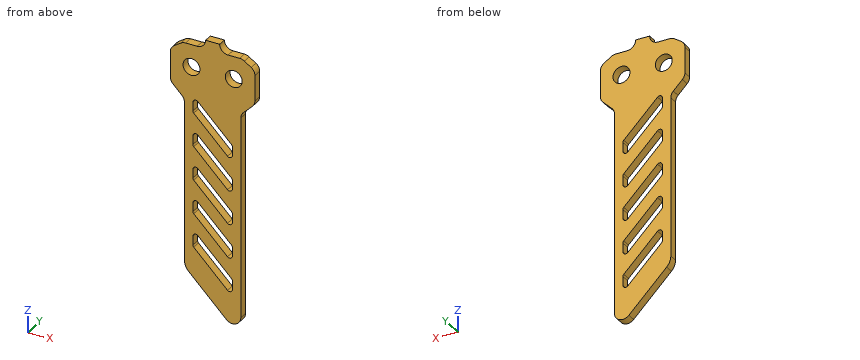
```python
from build123d import *
from OCP.BRepFilletAPI import BRepFilletAPI_MakeFillet

# Parameters (mm, degrees)
BOSS_EXTRUDE1_DEPTH     = 1.5
CUT_EXTRUDE1_DEPTH      = 105.097310244
CUT_EXTRUDE2_DEPTH      = 105.097310244
CUT_EXTRUDE2_DEPTH_BACK = 105.097310244
SKETCH2_R               = 3
FILLET1_R               = 3
FILLET2_R               = 3
FILLET3_R1              = 5
FILLET3_R2              = 3
FILLET4_R               = 1
LPATTERN1_COUNT         = 5
LPATTERN1_PITCH         = 12
FILLET4_OF_LPATTERN1_R  = 1


with BuildPart() as part:
    # Sketch1 → Boss-Extrude1 (new, symmetric)
    with BuildSketch(Plane(origin=(0, 0, 0), x_dir=(1, 0, 0), z_dir=(0, 1, 0))):
        Polygon((-10, 83), (10, 103), (10, 23), (15, 18), (15, 6), (10.5, 3), (2.5, 3), (2.5, 0), (-2.5, 0), (-2.5, 3), (-10.5, 3), (-15, 6), (-15, 18), (-10, 23), align=None)
    extrude(amount=BOSS_EXTRUDE1_DEPTH, both=True)

    # Sketch1<3> → Cut-Extrude1 (cut, symmetric)
    with BuildSketch(Plane(origin=(0, 0, 0), x_dir=(1, 0, 0), z_dir=(0, 1, 0))):
        Polygon((7, 89), (-7, 75), (-7, 69), (7, 83), align=None)
    cut_extrude1 = extrude(amount=CUT_EXTRUDE1_DEPTH, both=True, mode=Mode.SUBTRACT)

    # Sketch2 → Cut-Extrude2 (cut, two sides: drawn at the far end of the back side and taken through both)
    with BuildSketch(Plane(origin=(0, 0, 0), x_dir=(1, 0, 0), z_dir=(0, 1, 0)).offset(-CUT_EXTRUDE2_DEPTH_BACK)):
        with Locations(Location((-7.5, 11, 0), (0, 0, 270))):
            Circle(SKETCH2_R)
        with Locations(Location((7.5, 11, 0), (0, 0, 270))):
            Circle(SKETCH2_R)
    extrude(amount=CUT_EXTRUDE2_DEPTH + CUT_EXTRUDE2_DEPTH_BACK, mode=Mode.SUBTRACT)

    # Fillet1
    fillet1_edges = [part.edges().sort_by_distance(p)[0] for p in [
        (2.5, 0, -3),
        (-2.5, 0, -3),
    ]]
    fillet(fillet1_edges, radius=FILLET1_R - 0.0001)  # a hair under: the kernel refuses the full size

    # Fillet2
    fillet2_edges = [part.edges().sort_by_distance(p)[0] for p in [
        (-10, 0, -23),
        (-15, 0, -18),
        (-15, 0, -6),
        (-10.5, 0, -3),
        (10.5, 0, -3),
        (15, 0, -6),
        (15, 0, -18),
        (10, 0, -23),
    ]]
    fillet(fillet2_edges, radius=FILLET2_R)

    # Fillet3: one fillet with a radius per group of edges: ONE call of the kernel's fillet builder (fillet() takes one radius for all edges)
    fillet3_edges_1 = [part.edges().sort_by_distance(p)[0] for p in [
        (-10, 0, -83),
    ]]
    fillet3_edges_2 = [part.edges().sort_by_distance(p)[0] for p in [
        (10, 0, -103),
    ]]
    fillet3 = BRepFilletAPI_MakeFillet(part.part.solid().wrapped)
    for e in fillet3_edges_1:
        fillet3.Add(FILLET3_R1, e.wrapped)
    for e in fillet3_edges_2:
        fillet3.Add(FILLET3_R2, e.wrapped)
    add(Compound.cast(fillet3.Shape()), mode=Mode.REPLACE)

    # Fillet4
    fillet4_edges = [part.edges().sort_by_distance(p)[0] for p in [
        (-7, 0, -69),
        (-7, 0, -75),
        (7, 0, -89),
        (7, 0, -83),
    ]]
    fillet(fillet4_edges, radius=FILLET4_R)

    # LPattern1: Cut-Extrude1 ×5
    with Locations(*[(0, 0, i * LPATTERN1_PITCH) for i in range(1, LPATTERN1_COUNT)]):
        add(cut_extrude1, mode=Mode.SUBTRACT)

    # Fillet4 of LPattern1
    fillet4_of_lpattern1_edges = [part.edges().sort_by_distance(p)[0] for p in [
        (-7, 0, -57),
        (-7, 0, -63),
        (7, 0, -77),
        (7, 0, -71),
        (-7, 0, -45),
        (-7, 0, -51),
        (7, 0, -65),
        (7, 0, -59),
        (-7, 0, -33),
        (-7, 0, -39),
        (7, 0, -53),
        (7, 0, -47),
        (-7, 0, -21),
        (-7, 0, -27),
        (7, 0, -41),
        (7, 0, -35),
    ]]
    fillet(fillet4_of_lpattern1_edges, radius=FILLET4_OF_LPATTERN1_R)


solid = part.part
```
Build history of the part. All positions in model axes, mm. Round coordinates to 2 decimals unless told otherwise and drop trailing zeros. Order: outer loops, then holes, each group sorted by start corner. A loop starts at its lowest first (then second) coordinate and runs counter-clockwise, first axis right, second up. Notation, with made-up numbers: (45, -26.5) -> (69, -26.5) arc R23 ccw to (69, -3.5) -> close; hole circle Ø10 at (79.5, -27). An arc over 180 degrees is marked (long way). Answer in a Markdown table with one row per item.
1) Band-saw the part on D-D on y = -0.75. Give the number of separate pieces and of enclosed holes in the cut face, and give its area (3 significant figures).
Values:
| item | result |
|---|---|
| separate pieces | 1 |
| enclosed holes | 7 |
| area | 1,500 mm2 |
2) Band-saw the part on B-B on x = 1.25. Give the cut face in (y, z), and give its area (3 significant figures).
Values:
| item | result |
|---|---|
| outline | (-1.5, -94.25) -> (1.5, -94.25) -> (1.5, -83.25) -> (-1.5, -83.25) -> close; (-1.5, -77.25) -> (1.5, -77.25) -> (1.5, -71.25) -> (-1.5, -71.25) -> close; (-1.5, -65.25) -> (1.5, -65.25) -> (1.5, -59.25) -> (-1.5, -59.25) -> close; (-1.5, -53.25) -> (1.5, -53.25) -> (1.5, -47.25) -> (-1.5, -47.25) -> close; (-1.5, -41.25) -> (1.5, -41.25) -> (1.5, -35.25) -> (-1.5, -35.25) -> close; (-1.5, -29.25) -> (1.5, -29.25) -> (1.5, 0) -> (-1.5, 0) -> close |
| area | 193 mm2 |
3) Wall check: L1, parallel to X at y = -0.7, z = -11; L2, parallel to X at y = 1.2, z = -41.5; L3, parallel to X at y = 1.2, z = -9. Give the ranges that are in metal, low to high.
Values:
| item | result |
|---|---|
| L1 | -15 to -10.5, -4.5 to 4.5, 10.5 to 15 |
| L2 | -10 to -4.5, 1.5 to 10 |
| L3 | -15 to -9.74, -5.26 to 5.26, 9.74 to 15 |
4) Band-saw the part on A-A on z = -11. Give the cut face in (x, y), and give its area (3 significant figures).
Values:
| item | result |
|---|---|
| outline | (-15, -1.5) -> (-10.5, -1.5) -> (-10.5, 1.5) -> (-15, 1.5) -> close; (-4.5, -1.5) -> (4.5, -1.5) -> (4.5, 1.5) -> (-4.5, 1.5) -> close; (10.5, -1.5) -> (15, -1.5) -> (15, 1.5) -> (10.5, 1.5) -> close |
| area | 54.0 mm2 |
5) Band-saw the part on C-C on z = -68.5. Give the cut face in (x, y).
Values:
| item | result |
|---|---|
| outline | (-10, -1.5) -> (-1.5, -1.5) -> (-1.5, 1.5) -> (-10, 1.5) -> close; (4.5, -1.5) -> (10, -1.5) -> (10, 1.5) -> (4.5, 1.5) -> close |
6) Pin check, flat tips, straight feed: P1, Ø0.9, axis at x = 7, y = -0.5, coming from the +Z side; P2, Ø0.9, axis at y = 0.5, z = -60.5, coming from the +X side; P3, Ø9.5, axis at x = 7.5, z = -11, coming from the -Y side; P4, Ø0.9, axis at y = 0.5, z = -61, coming from the -X side. Stop position of each tip, or through.
Values:
| item | result |
|---|---|
| P1 | z = -3 |
| P2 | x = 10 |
| P3 | y = -1.5 |
| P4 | x = -10 |
